from build123d import *

# Parameters (mm, degrees)
SKETCH2_R          = 0.35
CUT_EXTRUDE1_DEPTH = 5


with BuildPart() as part:
    # Sketch1 → Revolve1 (revolve)
    with BuildSketch(Plane.XY, mode=Mode.PRIVATE) as revolve1_sk:
        Polygon((0, 0), (3, 0), (3, 1.5), (2.5, 1.5), (2.5, 48.5), (3, 48.5), (3, 50), (0, 50), align=None)
    revolve(revolve1_sk.sketch.rotate(Axis((0, 50, 0), (0, -1, 0)), 180), axis=Axis((0, 50, 0), (0, -1, 0)))

    # Sketch2 → Cut-Extrude1 (cut, symmetric)
    with BuildSketch(Plane.XY):
        with Locations(Location((0, 0.802923523, 0), (0, 0, 180))):
            Circle(SKETCH2_R)
    extrude(amount=CUT_EXTRUDE1_DEPTH, both=True, mode=Mode.SUBTRACT)


solid = part.part
For this review, take the finished solid that the model builds, in its own axes (mm). A direction names the side the tool comes from. Give positions to 0.01 mm unless a question says otherwise; leave off trailing zeros. Loops run counter-clockwise (first coordinate to the right, second up) from the corner with the lowest first, then second, coordinate; pieces in that order, holes last. Notation, with made-up numbers: M 39,19.5 L 46,19.5 A18 cw 46,50.5 Z; hole C 40.25,44.5 d4. An arc over 180 degrees is marked long. Answer as a JSON object with one key per item and string values. Group by question number.
Q1. Mouldability with a two-part tool opening along Y and no side actions: class faces 1 (the cylindrical face through (-2.86, 49.26, -0.9)), 2 (the flat face through (-2, 48.5, -2)), 3 (the flat face through (0, 0, 0)), 4 (the flat face through (0, 50, 0)) as +Y half, -Y half, draft (parallel to the pull), parting line (faces both ways), or undercut.
Q2. Tool access review of faces 5 (the cylindrical face through (-2.86, 0.76, -0.9)), 6 (the cylindrical face through (2.5, 25.3, -0.1)): name each direction out of +Z, -Z, +X, -X, +Y, -Y from which nothing blocks a thin tool from reaching the whole face with its end or side.
Q3. Insertion check: P1, Ø2, axis at y = 34, z = -2, coming from the +X side; P2, Ø1.5, axis at y = 16.5, z = -1, coming from the -X side. Each pin has a flat end and moves straight along its axis. Give the tip position at first contact, or say it passes through.
Q4. Add section A-A on z = 1.5. Give the boundary of the cut face in (x, y), and give its area (3 significant figures).
Q5. Add section C-C on x = 1. Give the boundary of the cut face in (y, z), and give its area (3 significant figures).
Q6. Add section B-B on y = 25.5. Give the boundary of the cut face in (x, z), and give its area (3 significant figures).
Q7. For probe 1 along Y at (x, z) = (-0.5, 2.5); probe 2 along Y at (x, z) = (0, 1); probe 3 along Z at (x, y) = (0, 28), list the stretches that pass through material, from the lowest coordinate up. Write a range as [from, to].
Checked values:
{
 "1": {"face 1": "draft", "face 2": "undercut", "face 3": "-Y half", "face 4": "+Y half"},
 "2": {"face 5": "+Y, -Y", "face 6": "none"},
 "3": {"P1": "x = 2.29", "P2": "x = -2.49"},
 "4": {"outline": "M -2.6,0 L 2.6,0 L 2.6,1.5 L 2,1.5 L 2,48.5 L 2.6,48.5 L 2.6,50 L -2.6,50 L -2.6,48.5 L -2,48.5 L -2,1.5 L -2.6,1.5 Z; hole C 0,0.8 d0.7", "area": "203 mm²"},
 "5": {"outline": "M 0,-2.83 L 1.5,-2.83 L 1.5,-2.29 L 48.5,-2.29 L 48.5,-2.83 L 50,-2.83 L 50,2.83 L 48.5,2.83 L 48.5,2.29 L 1.5,2.29 L 1.5,2.83 L 0,2.83 Z", "area": "232 mm²"},
 "6": {"outline": "C 0,0 d5", "area": "19.6 mm²"},
 "7": {"probe 1": "[0, 1.5], [48.5, 50]", "probe 2": "[0, 0.45], [1.15, 50]", "probe 3": "[-2.5, 2.5]"}
}
